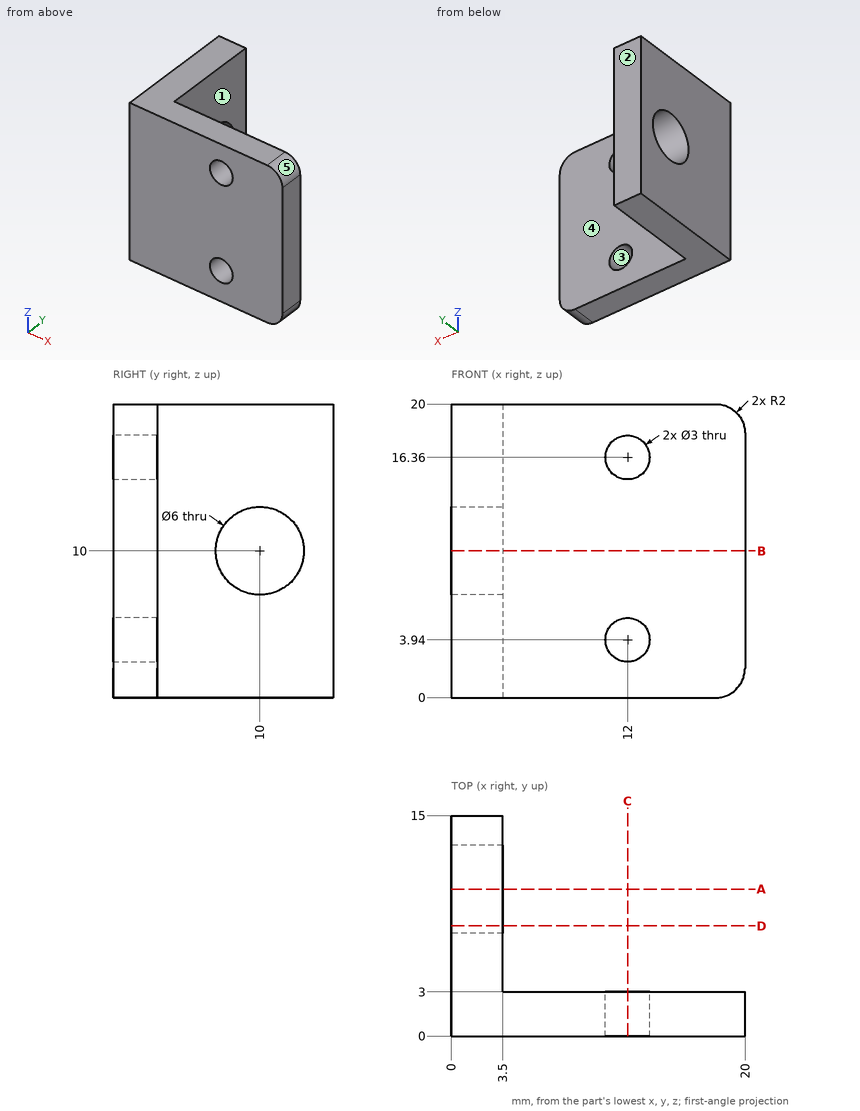
Geometry: see drawing. Coordinates: mm, zero at the bounding-box minimum. A direction names the side the tool comes from. Coordinates: 2 decimals unless noted, no trailing zeros. Loops run counter-clockwise (first coordinate to the right, second up) from the corner with the lowest first, then second, coordinate; pieces in that order, holes last.
(1) Section D-D on y = 7.5. Return the cut outline in (x, z), then the cut area to 3 significant figures.
(2) Material intervals for probe 1 along X at (y, z) = (11, 7); probe 2 along Y at (x, z) = (17, 14.5); probe 3 along Z at (x, y) = (1.5, 9), sorted ascending.
(3) Section C-C on x = 12. Return the cut outline in (y, z).
(4) Pull-direction query (X, two-part tool) for the marked faces 1, 2 and 3; classes: released by +X, released by -X, zero draft, split by the parting line, or undercut.
(5) Section B-B on z = 10. Return the cut outline in (x, y).
(6) First-contact query: pin 1 Ø8 at (x, z) = (8.5, 13) entering from +Y; pin 2 Ø6 at (y, z) = (7.5, 8) entering from +X; pin 3 Ø2.5 at (x, z) = (12, 16.36) entering from -Y. Flat tips, straight axial feed; report the tip coordinate or a pass-through.
(7) Set-up query: the marked faces 4 and 5. Return all of +Z, -Z, +X, -X, +Y, -Y with unobstructed straight access to the full face (end or side cutting, diameter ignored); none if empty.
(8) Section A-A on y = 10. Return the cut outline in (x, z), then the cut area to 3 significant figures.
Data:
1. outline: (0, 0) - (3.5, 0) - (3.5, 8.34) - (0, 8.34) - close; (0, 11.66) - (3.5, 11.66) - (3.5, 20) - (0, 20) - close
1. area: 58.4 mm2
2. probe 1: x = 0 to 3.5
2. probe 2: y = 0 to 3
2. probe 3: z = 0 to 7.17, 12.83 to 20
3. outline: (0, 0) - (3, 0) - (3, 2.44) - (0, 2.44) - close; (0, 5.44) - (3, 5.44) - (3, 14.86) - (0, 14.86) - close; (0, 17.86) - (3, 17.86) - (3, 20) - (0, 20) - close
4. face 1: released by +X
4. face 2: zero draft
4. face 3: undercut
5. outline: (0, 0) - (20, 0) - (20, 3) - (3.5, 3) - (3.5, 7) - (0, 7) - close; (0, 13) - (3.5, 13) - (3.5, 15) - (0, 15) - close
6. pin 1: stops at y = 3
6. pin 2: stops at x = 3.5
6. pin 3: passes through
7. face 4: +Z, -Z, +X, +Y
7. face 5: +Z, +X, +Y, -Y
8. outline: (0, 0) - (3.5, 0) - (3.5, 7) - (0, 7) - close; (0, 13) - (3.5, 13) - (3.5, 20) - (0, 20) - close
8. area: 49.0 mm2
